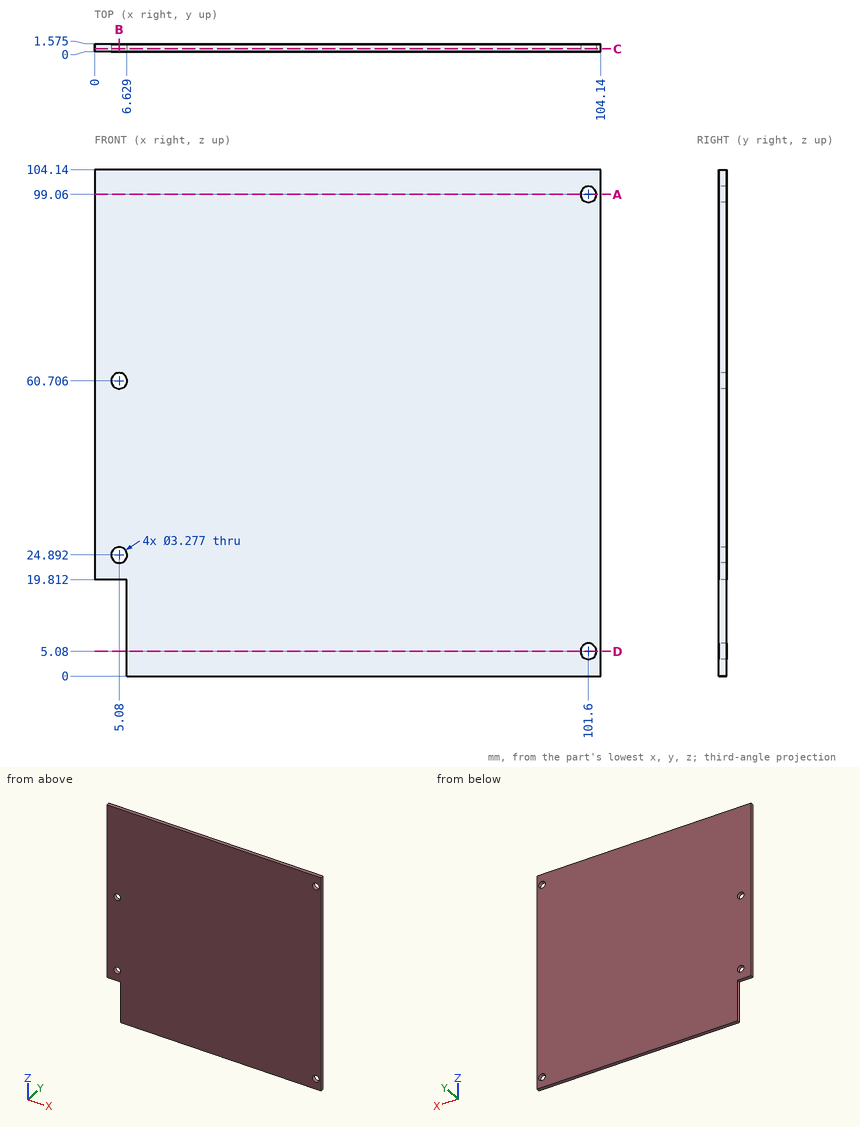
Input: dimensioned drawing with shaded views. Units: mm. Origin: part minimum x, y, z. Round coordinates to 2 decimals unless told otherwise and drop trailing zeros. Order: outer loops, then holes, each group sorted by start corner. A loop starts at its lowest first (then second) coordinate and runs counter-clockwise, first axis right, second up. Notation, with made-up numbers: (81.5, -25.5) -> (123.5, -25.5) arc R25 ccw to (123.5, -4.5) -> close; hole circle Ø9 at (55, 70). An arc over 180 degrees is marked (long way). One line per item, written item: value. Start each with the question number.
Q1. Section query B-B (x = 5.08). Return the cut outline in (y, z) (1 decimal).
Q2. Section query A-A (z = 99.06). Return the cut outline in (x, y) (1 decimal), plus the area to 3 significant figures.
Q3. Material intervals for probe 1 along Z at (x, y) = (101.6, 1); probe 2 along Z at (x, y) = (5.08, 1) (1 decimal); probe 3 along X at (y, z) = (0.45, 61), sorted ascending.
Q4. Section query C-C (y = 0.55). Return the cut outline in (x, z) (1 decimal).
Q5. Section query D-D (z = 5.08). Return the cut outline in (x, y) (1 decimal).
Q6. Pin query (flat end, axial travel): pin 1 (0.5 mm diameter, centred on x = 4, y = 0.5, fed in from -Z); pin 2 (2.5 mm diameter, centred on x = 5.08, z = 60.706, fed in from -Y). Return the tip coordinate at first contact, or that it passes through.
Findings below:
1. outline: (0, 19.8) -> (1.6, 19.8) -> (1.6, 23.3) -> (0, 23.3) -> close; (0, 26.5) -> (1.6, 26.5) -> (1.6, 59.1) -> (0, 59.1) -> close; (0, 62.3) -> (1.6, 62.3) -> (1.6, 104.1) -> (0, 104.1) -> close
2. outline: (0, 0) -> (100, 0) -> (100, 1.6) -> (0, 1.6) -> close; (103.2, 0) -> (104.1, 0) -> (104.1, 1.6) -> (103.2, 1.6) -> close
2. area: 159 mm²
3. probe 1: 0 to 3.44, 6.72 to 97.42, 100.7 to 104.14
3. probe 2: 19.8 to 23.3, 26.5 to 59.1, 62.3 to 104.1
3. probe 3: 0 to 3.47, 6.69 to 104.14
4. outline: (0, 19.8) -> (6.6, 19.8) -> (6.6, 0) -> (104.1, 0) -> (104.1, 104.1) -> (0, 104.1) -> close; hole circle Ø3.3 at (5.1, 24.9); hole circle Ø3.3 at (5.1, 60.7); hole circle Ø3.3 at (101.6, 5.1); hole circle Ø3.3 at (101.6, 99.1)
5. outline: (6.6, 0) -> (100, 0) -> (100, 1.6) -> (6.6, 1.6) -> close; (103.2, 0) -> (104.1, 0) -> (104.1, 1.6) -> (103.2, 1.6) -> close
6. pin 1: z = 19.81
6. pin 2: through
